from build123d import *

# Parameters (mm, degrees)
F0_W      = 146.05
F0_H      = 76.2
F1_DEPTH  = 9.031111
F2_R      = 7.62
F3_W      = 8.543316
F3_H      = 2.313646
F4_DEPTH  = 25.4
F5_R      = 2.068187
F6_DEPTH  = 2.54
F7_DEPTH  = 38.1
F8_W      = 114.3
F8_H      = 70.64375
F9_DEPTH  = 1.27
F10_R     = 2.211011
F10_R_2   = 1.499171
F10_R_3   = 1.566639
F10_R_4   = 1.611216
F10_R_5   = 2.610704
F10_R_6   = 1.480203
F10_W     = 2.047286
F10_H     = 9.729784
F10_W_2   = 1.917139
F10_H_2   = 10.160214
F11_DEPTH = 1.27
F12_R     = 4.643642
F12_R_2   = 2.536257
F12_R_3   = 4.132051
F13_DEPTH = 1.27


with BuildPart() as f1:
    # F0 (on Top) → F1 (new body)
    with BuildSketch(Plane.XY):
        with Locations((2.936147, 0.115003)):
            Rectangle(F0_W, F0_H)
    extrude(amount=F1_DEPTH)

    # F2
    f2_edges = [f1.edges().sort_by_distance(p)[0] for p in [
        (75.961147, -37.984997, 4.515556),
        (-70.088853, -37.984997, 4.515556),
        (-70.088853, 38.215003, 4.515556),
        (75.961147, 38.215003, 4.515556),
    ]]
    fillet(f2_edges, radius=F2_R)

    # F3 (on face) → F4 (cut)
    with BuildSketch(Plane.YZ.offset(75.961147)):
        with Locations((0, 3.654829)):
            Rectangle(F3_W, F3_H)
    extrude(amount=-F4_DEPTH, mode=Mode.SUBTRACT)

    # F5 (on face) → F6 (cut)
    with BuildSketch(Plane(origin=(-70.088853, 0, 0), x_dir=(0, -1, 0), z_dir=(-1, 0, 0))):
        with Locations((-21.835269, 4.515556)):
            Circle(F5_R)
    extrude(amount=-F6_DEPTH, mode=Mode.SUBTRACT)

    # F5 (on face) → F7 (cut)
    with BuildSketch(Plane(origin=(-70.088853, 0, 0), x_dir=(0, -1, 0), z_dir=(-1, 0, 0))):
        with Locations((-21.835269, 4.515556)):
            Circle(F5_R)
    extrude(amount=-F7_DEPTH, mode=Mode.SUBTRACT)

    # F8 (on face) → F9 (cut)
    with BuildSketch(Plane.XY.offset(9.031111)):
        with Locations((-2.620103, -0.281872)):
            Rectangle(F8_W, F8_H)
    extrude(amount=-F9_DEPTH, mode=Mode.SUBTRACT)

    # F10 (on face) → F11 (cut)
    with BuildSketch(Plane.XY.offset(9.031111)):
        with Locations((-64.550646, 26.395293)):
            Circle(F10_R)
        with Locations((-64.775102, 20.281654)):
            Circle(F10_R_2)
        with Locations((71.801327, 26.097044)):
            Circle(F10_R_3)
        with Locations((71.801327, -25.825897)):
            Circle(F10_R_4)
        with Locations((-64.420246, -29.946957)):
            Circle(F10_R_5)
        with Locations((-64.775102, -24.518941)):
            Circle(F10_R_6)
        Polygon((-63.610494, 16.045377), (-65.666994, 16.045377), (-65.712694, -19.34428), (-63.610494, -19.34428), align=None)
        with Locations((72.82497, 17.815223)):
            Rectangle(F10_W, F10_H)
        with Locations((72.759896, -16.931376)):
            Rectangle(F10_W_2, F10_H_2)
    extrude(amount=-F11_DEPTH, mode=Mode.SUBTRACT)

    # F12 (on face) → F13 (cut)
    with BuildSketch(Plane(origin=(0, 0, 0), x_dir=(1, 0, 0), z_dir=(0, 0, -1))):
        with Locations((-57.045136, 0)):
            Circle(F12_R)
        with Locations((-46.850082, 0)):
            Circle(F12_R_2)
        with Locations((-32.002568, 0)):
            Circle(F12_R_3)
    extrude(amount=-F13_DEPTH, mode=Mode.SUBTRACT)


solid = f1.part
Work out the finished part from the listing and answer in its coordinate system (mm). A direction names the side the tool comes from. Round coordinates to 2 decimals unless told otherwise and drop trailing zeros. Write each loop counter-clockwise with the first axis right and the second up, starting at its lowest first coordinate (ties: lowest second). Pieces come first, ordered by that corner, then holes. Notation, with made-up numbers: (23.25, 87) -> (52.25, 87) arc R27 ccw to (52.25, 105) -> close; hole circle Ø1 at (22, 68). An arc over 180 degrees is marked (long way). Answer as CSV lines item,"result". Start each with the question number.
(1) The part is cut by section A-A, the plane y = -18. Give the vertices of the cut face in (x, z), then the cut area to 3 significant figures.
(2) Each of these flat-tipped pins is pushed along its axis until it touches: pin 1 (5 mm diameter, centred on x = 14, y = 26.5, fed in from +Z); pin 2 (6.5 mm diameter, centred on x = -32, y = 0, fed in from -Z). Where does it stop, or does it pass through?
(3) The part is cut by section B-B, the plane x = 36. Give the vertices of the cut face in (y, z) (3 decimals), then the cut area to 3 significant figures.
(4) Find the intervals of material crossed by probe 1 along X at (y, z) = (-6, 8.75); probe 2 along X at (y, z) = (0, 1.05); probe 3 along Y at (x, z) = (-20, 8) (3 decimals), in increasing order.
(5) The part is cut by section C-C, the plane y = 0. Give the vertices of the cut face in (x, z), then the cut area to 3 significant figures.
(6) The mould has two halves that part along Z. Classify faces 1 (the flat face through (-47, 0, 1.27)), 2 (the flat face through (63, 0, 4.812)), 3 (the cylindrical face through (-51.306, 19.925, 3.723)), 4 (the cylindrical face through (-67.92, 35.92, 4.58)): +Z half, -Z half, draft (parallel to the pull), parting line (faces both ways), or undercut.
(7) A tool of negligible diameter and unlimited length cuts with its end or side. For faces 5 (the cylindrical face through (72.524, 24.707, 8.405)), 6 (the cylindrical face through (-44.43, -0.76, 0.63)), 7 (the flat face through (63, 0, 2.498)), from which of +Z, -Z, +X, -X, +Y, -Y can it reach the whole face along a straight path? Write none if from no direction.
Output values:
1,outline,"(-70.09, 0) -> (75.96, 0) -> (75.96, 9.03) -> (73.72, 9.03) -> (73.72, 7.76) -> (71.8, 7.76) -> (71.8, 9.03) -> (54.53, 9.03) -> (54.53, 7.76) -> (-59.77, 7.76) -> (-59.77, 9.03) -> (-63.61, 9.03) -> (-63.61, 7.76) -> (-65.71, 7.76) -> (-65.71, 9.03) -> (-70.09, 9.03) -> close"
1,area,"1,170 mm²"
2,pin 1,"stops at z = 7.76"
2,pin 2,"stops at z = 1.27"
3,outline,"(-37.985, 0) -> (38.215, 0) -> (38.215, 9.031) -> (35.04, 9.031) -> (35.04, 7.761) -> (-35.604, 7.761) -> (-35.604, 9.031) -> (-37.985, 9.031) -> close"
3,area,"598 mm²"
4,probe 1,"x = -70.09 to -65.7, -63.61 to -59.77, 54.53 to 75.96"
4,probe 2,"x = -70.09 to -61.69, -52.4 to -49.39, -44.31 to -36.13, -27.87 to 75.96"
4,probe 3,"y = -37.985 to -35.604, 35.04 to 38.215"
5,outline,"(-70.09, 0) -> (-61.69, 0) -> (-61.69, 1.27) -> (-52.4, 1.27) -> (-52.4, 0) -> (-49.39, 0) -> (-49.39, 1.27) -> (-44.31, 1.27) -> (-44.31, 0) -> (-36.13, 0) -> (-36.13, 1.27) -> (-27.87, 1.27) -> (-27.87, 0) -> (75.96, 0) -> (75.96, 2.5) -> (50.56, 2.5) -> (50.56, 4.81) -> (75.96, 4.81) -> (75.96, 9.03) -> (54.53, 9.03) -> (54.53, 7.76) -> (-59.77, 7.76) -> (-59.77, 9.03) -> (-63.61, 9.03) -> (-63.61, 7.76) -> (-65.69, 7.76) -> (-65.69, 9.03) -> (-70.09, 9.03) -> close"
5,area,"1,080 mm²"
6,face 1,"-Z half"
6,face 2,"undercut"
6,face 3,"undercut"
6,face 4,"draft"
7,face 5,"+Z"
7,face 6,"-Z"
7,face 7,"+X"
